from build123d import *

# Parameters (mm, degrees)
F1_DEPTH      = 12
F3_DEPTH      = 2.5
F5_DEPTH      = 25
F6_R          = 30
F8_DEPTH      = 25
F8_DEPTH_BACK = 25
F9_R          = 4
F10_DEPTH     = 25
F11_R         = 1.8
F12_DEPTH     = 7.5
F13_SIZE      = 0.75
F14_SIZE      = 0.75
F15_SIZE      = 0.75
F16_W         = 5
F16_H         = 50.1374751329
F17_DEPTH     = 3
F18_R         = 2.49999


# Not quite as in the source:
# - a fillet or chamfer is up to 0.001 mm smaller than in the source, because OpenCascade refuses the exact size


with BuildPart() as f1:
    # F0 (on Top) → F1 (new body)
    with BuildSketch(Plane.XY):
        with BuildLine():
            Line((-3.74e-08, 99.6128183121), (0, 0))
            ThreePointArc((0, 0), (18.500000007, -18.499999993), (37, 1.39e-08))
            Line((37, 1.39e-08), (36.9999999626, 99.6128183121))
            Line((36.9999999626, 99.6128183121), (47.8017579937, 148.7838923931))
            Line((47.8017579937, 148.7838923931), (47.8017579937, 159.1853948904))
            Line((47.8017579937, 159.1853948904), (34.9798792017, 159.1853948904))
            ThreePointArc((34.9798792017, 159.1853948904), (2.004546746, 159.6126733438), (34.9234827971, 161.5872028336))
            Line((34.9234827971, 161.5872028336), (47.8017579834, 161.5872028336))
            Line((47.8017579834, 161.5872028336), (47.8017578313, 168.1936387276))
            Line((47.8017578313, 168.1936387276), (42.1191508, 168.1936387276))
            ThreePointArc((42.1191508, 168.1936387276), (13.0001519828, 184.387531079), (-6.3497242683, 157.2629936512))
            Line((-6.3497242683, 157.2629936512), (-3.74e-08, 99.6128183121))
        make_face()
    extrude(amount=F1_DEPTH)

    # F2 (on face) → F3 (join)
    with BuildSketch(Plane(origin=(0, 0, 0), x_dir=(1, 0, 0), z_dir=(0, 0, -1))):
        with BuildLine():
            ThreePointArc((29.3, -7e-09), (18.5, 10.799999993), (7.7, -7e-09))
            Line((7.7, -7e-09), (7.7, -72.500000007))
            ThreePointArc((7.7, -72.500000007), (18.5, -83.300000007), (29.3, -72.500000007))
            Line((29.3, -72.500000007), (29.3, -7e-09))
        make_face()
    extrude(amount=F3_DEPTH)

    # F4 (on face) → F5 (cut)
    with BuildSketch(Plane(origin=(0, 0, -2.5), x_dir=(1, 0, 0), z_dir=(0, 0, -1))):
        with BuildLine():
            ThreePointArc((21.75, 4.749999993), (18.5, 7.999999993), (15.25, 4.749999993))
            Line((15.25, 4.749999993), (15.25, -77.250000007))
            ThreePointArc((15.25, -77.250000007), (18.5, -80.500000007), (21.75, -77.250000007))
            Line((21.75, -77.250000007), (21.75, 4.749999993))
        make_face()
    extrude(amount=-F5_DEPTH, mode=Mode.SUBTRACT)

    # F6
    f6_edges = [f1.edges().sort_by_distance(p)[0] for p in [
        (0, 99.612818, 6),
        (37, 99.612818, 6),
    ]]
    fillet(f6_edges, radius=F6_R)

    # F7 (on face) → F8 (cut, two sides)
    with BuildSketch(Plane(origin=(0, 168.1936387276, 0), x_dir=(-1, 0, 0), z_dir=(0, 1, 0))) as f8_sk:
        with BuildLine():
            ThreePointArc((-42.1191508, 4.5), (-41.0584906283, 4.9393398282), (-40.6191508, 6))
            ThreePointArc((-40.6191508, 6), (-41.0584906283, 7.0606601718), (-42.1191508, 7.5))
            Line((-42.1191508, 7.5), (-42.1191508, 4.5))
        make_face()
        with BuildLine():
            Line((-42.1191508, 4.5), (-42.1191508, 7.5))
            ThreePointArc((-42.1191508, 7.5), (-43.6191508, 6), (-42.1191508, 4.5))
        make_face()
    extrude(amount=-F8_DEPTH, mode=Mode.SUBTRACT)
    extrude(f8_sk.sketch, amount=F8_DEPTH_BACK, mode=Mode.SUBTRACT)

    # F9 (on face) → F10 (cut)
    with BuildSketch(Plane(origin=(0, 168.1936387276, 0), x_dir=(-1, 0, 0), z_dir=(0, 1, 0))):
        with Locations((-42.1191508, 6)):
            Circle(F9_R)
    extrude(amount=F10_DEPTH, mode=Mode.SUBTRACT)

    # F11 (on face) → F12 (cut)
    with BuildSketch(Plane(origin=(0, 168.1936387276, 0), x_dir=(-1, 0, 0), z_dir=(0, 1, 0))):
        with Locations((-42.1191508, 6)):
            Circle(F11_R)
    extrude(amount=-F12_DEPTH, mode=Mode.SUBTRACT)

    # F13
    f13_edges = [f1.edges().sort_by_distance(p)[0] for p in [
        (37, 48.178243, 12),
        (41.390819, 159.185395, 12),
        (2.004547, 159.612673, 12),
        (47.801758, 153.984644, 12),
    ]]
    chamfer(f13_edges, length=F13_SIZE)

    # F14
    f14_edges = [f1.edges().sort_by_distance(p)[0] for p in [
        (2.004547, 159.612673, 0),
    ]]
    chamfer(f14_edges, length=F14_SIZE)

    # F15
    f15_edges = [f1.edges().sort_by_distance(p)[0] for p in [
        (42.75022, 125.788603, 0),
        (13.000152, 184.387531, 0),
        (-3.265028, 129.256533, 0),
        (37.175182, 99.593803, 0),
        (-0.045117, 99.610341, 0),
        (37, 48.178243, 0),
        (0, 48.982832, 0),
        (18.5, -18.5, 0),
    ]]
    chamfer(f15_edges, length=F15_SIZE)

    # F16 (on face) → F17 (cut)
    with BuildSketch(Plane(origin=(0, 0, 0), x_dir=(1, 0, 0), z_dir=(0, 0, -1))):
        with Locations((25, -111.8474081159)):
            Rectangle(F16_W, F16_H)
        with Locations((12, -111.8474081159)):
            Rectangle(F16_W, F16_H)
    extrude(amount=-F17_DEPTH, mode=Mode.SUBTRACT)

    # F18 (radius 2.5 in the source; OpenCascade refuses exactly that, so slightly less here)
    f18_edges = [f1.edges().sort_by_distance(p)[0] for p in [
        (22.5, 136.916146, 1.5),
        (27.5, 136.916146, 1.5),
        (14.5, 136.916146, 1.5),
        (9.5, 136.916146, 1.5),
        (9.5, 86.778671, 1.5),
        (14.5, 86.778671, 1.5),
        (27.5, 86.778671, 1.5),
        (22.5, 86.778671, 1.5),
    ]]
    fillet(f18_edges, radius=F18_R)


solid = f1.part
Could you check a few things on this model? Use its own coordinates, in mm. A direction names the side the tool comes from. Give positions to 0.01 mm unless a question says otherwise; leave off trailing zeros. Order: outer loops, then holes, each group sorted by start corner. A loop starts at its lowest first (then second) coordinate and runs counter-clockwise, first axis right, second up.
1. For faces 1 (the flat face through (12, 111, 3)), 2 (the flat face through (42.7, 127.2, 0.4)), 3 (the flat face through (-2.94, 129.69, 0.38)), 4 (the flat face through (37, 48, 6)), 5 (the cylindrical face through (43.917, 164.937, 6.079)), which set-ups out of +Z, -Z, +X, -X, +Y, -Y let a thin tool reach every point of the face, with its end or its side?
2. Suppose I cut it at C-C (y = 115). List the corners of the cut face in (x, z) for me.
3. Will these pins go through, and if not, where does the flat tip stop? P1, Ø1.5, axis at x = 11, y = 113.5, coming from the -Z side; P2, Ø0.9, axis at y = 102, z = 1.5, coming from the -X side; P3, Ø1, axis at x = 33, z = 5.5, coming from the +Y side.
4. We'd pull the mould along Y, two halves only. Please class faces 6 (the conical face through (1.915, 158.931, 11.37)), 7 (the flat face through (-2.94, 129.69, 11.62)), 8 (the cylindrical face through (18.4, 80.5, 4.6)), 9 (the cylindrical face through (18.3, 83.3, -1.2)): pulls with the +Y half, pulls with the -Y half, needs draft (parallel to the pull), parting line crosses it, or undercut.
5. Suppose I cut it at B-B (y = 44). List the corners of the cut face in (x, z) for me, plus the area to 3 significant figures.
6. I need wall thicknesses on L1, parallel to Y at x = 18.5, z = 5.75; L2, parallel to X at y = 96, z = 1.25; L3, parallel to X at y = 28, z = 1.75. Which ranges of each line are inside material? Lowest first, please.
7. Suppose I cut it at A-A (x = 18.5). List the corners of the cut face in (y, z) for me.
Solved:
1. face 1: -Z
1. face 2: -Z, +X, -Y
1. face 3: -Z, -X, -Y
1. face 4: +Z, -Z, +X, -Y
1. face 5: +Y
2. outline: (-1.69, 0.75) - (-0.94, 0) - (9.5, 0) - (9.5, 3) - (14.5, 3) - (14.5, 0) - (22.5, 0) - (22.5, 3) - (27.5, 3) - (27.5, 0) - (39.61, 0) - (40.38, 0.75) - (40.38, 11.25) - (39.61, 12) - (-0.94, 12) - (-1.69, 11.25) - close
3. P1: stops at z = 3
3. P2: stops at x = -0.31
3. P3: stops at y = 180.71
4. face 6: undercut
4. face 7: pulls with the -Y half
4. face 8: undercut
4. face 9: pulls with the +Y half
5. outline: (0, 0.75) - (0.75, 0) - (7.7, 0) - (7.7, -2.5) - (15.25, -2.5) - (15.25, 12) - (0.75, 12) - (0, 11.25) - close; (21.75, -2.5) - (29.3, -2.5) - (29.3, 0) - (36.25, 0) - (37, 0.75) - (37, 11.25) - (36.25, 12) - (21.75, 12) - close
5. area: 403 mm2
6. L1: y = -18.5 to -8, 80.5 to 143.5, 176.5 to 185
6. L2: x = 0 to 9.5, 14.5 to 22.5, 27.5 to 37
6. L3: x = 0 to 15.25, 21.75 to 37
7. outline: (-18.5, 0.75) - (-17.75, 0) - (-10.8, 0) - (-10.8, -2.5) - (-8, -2.5) - (-8, 12) - (-17.75, 12) - (-18.5, 11.25) - close; (80.5, -2.5) - (83.3, -2.5) - (83.3, 0) - (142.75, 0) - (143.5, 0.75) - (143.5, 11.25) - (142.75, 12) - (80.5, 12) - close; (176.5, 0.75) - (177.25, 0) - (184.25, 0) - (185, 0.75) - (185, 11.25) - (184.25, 12) - (177.25, 12) - (176.5, 11.25) - close
